Read the model definition and answer for the solid it produces. Units are mm, in the model's axes. A direction names the side the tool comes from. Coordinates: 2 decimals unless noted, no trailing zeros. Write each loop counter-clockwise with the first axis right and the second up, starting at its lowest first coordinate (ties: lowest second). Pieces come first, ordered by that corner, then holes. Notation, with made-up numbers: M -30.75,45 L 3.25,45 A18 cw 3.25,60 Z; hole C -26,20 d2. An arc over 180 degrees is marked long. Use a Markdown table: item, result. Add a question column.
Autodesk Inventor part; units mm, degrees
ref_plane "YZ Plane" through (0, 0, 0) normal (1, 0, 0) x (0, 1, 0)
ref_plane "XZ Plane" through (0, 0, 0) normal (0, 1, 0) x (-1, 0, 0)
ref_plane "XY Plane" through (0, 0, 0) normal (0, 0, 1) x (1, 0, 0)
sketch "Sketch1" plane through (0, 0, 0) normal (0, 1, 0) x (-1, 0, 0)
  line L0 (0, -3) -> (-0.5, -3)
  line L1 (-0.5, -3) -> (-0.5, -4.2634)
  line L2 (-0.5, -4.2634) -> (-0.5134, -4.2634)
  line L3 (-0.5134, -4.2634) -> (-4.9134, -3)
  line L4 (0, -3) -> (0, 0)
  line L5 (-4.9134, -3) -> (-4.9134, 0)
  line L6 (0, 0) -> (-4.9134, 0) construction
  line L7 (0, 3) -> (-0.5, 3)
  line L8 (-0.5, 3) -> (-0.5, 4.2634)
  line L9 (-0.5, 4.2634) -> (-0.5134, 4.2634)
  line L10 (-0.5134, 4.2634) -> (-4.9134, 3)
  line L11 (0, 3) -> (0, 0)
  line L12 (-4.9134, 3) -> (-4.9134, 0)
  dimension "d0" = 6
  dimension "d1" = 0.5
  dimension "d4" = 4.4
extrude "Extrusion1" add sketch "Sketch1" along normal blind 10
sketch "Sketch2" plane through (0, 0, -3) normal (-1, 0, 0) x (0, 0, 1)
  line L0 (3, 0) -> (3, 10) construction
  line L1 (0, 10) -> (6, 10)
  point P0 (3, 5)
hole "Hole2" at (0, 5, 0) direction (1, 0, 0) diameter 4.134 end through all
properties part number "m5_t_nut"
Item 1: Find section D-D on x = 1.85. Give the vertices of the cut face in (y, z), then the cut area to 3 significant figures.
Item 2: Each of these flat-tipped pins is pushed along its axis until it touches: pin 1 (0.6 mm diameter, centred on x = 0, y = 4.5, fed in from -Z); pin 2 (1.4 mm diameter, centred on y = 7, z = 4, fed in from -X); pin 3 (3.5 mm diameter, centred on y = 5, z = 0, fed in from +X). Where does it stop, or does it pass through?
Item 3: For faces 1 (the flat face through (0.5, 5, -4)), 2 (the flat face through (2.68, 4.93, 3.64)), 3 (the flat face through (0.5, 5, 4)), determine the directions among +Z, -Z, +X, -X, +Y, -Y from which every point of the face is accessible in a straight line to the end or side of a thin tool.
Item 4: Consider probe 1 along Y at (x, z) = (3.75, 0); probe 2 along Z at (x, y) = (0.4, 5.25); probe 3 along Z at (x, y) = (2.45, 5). Determine where each line is inside the solid, lowest interval first.
Item 5: Determine the mould class of faces 4 (the cylindrical face through (2.49, 2.95, -0.27)), 5 (the flat face through (0, 2.7, 0)), 6 (the flat face through (2, 0, 0)), 7 (the flat face through (2, 10, 0)) for opening direction Y: pulls with the +Y half, pulls with the -Y half, needs draft (parallel to the pull), parting line crosses it, or undercut.
Item 6: Find section B-B on z = 0. Give the vertices of the cut face in (x, y), then the cut area to 3 significant figures.
Geometry says:
| question | item | result |
|---|---|---|
| 1 | outline | M 0,-3.88 L 10,-3.88 L 10,3.88 L 0,3.88 Z; hole C 5,0 d4.13 |
| 1 | area | 64.2 mm2 |
| 2 | pin 1 | stops at z = -3 |
| 2 | pin 2 | stops at x = 0.5 |
| 2 | pin 3 | passes through |
| 3 | face 1 | -Z, -X, +Y, -Y |
| 3 | face 2 | +Z, +X, +Y, -Y |
| 3 | face 3 | +Z, -X, +Y, -Y |
| 4 | probe 1 | y = 0 to 2.93, 7.07 to 10 |
| 4 | probe 2 | z = -3 to -2.05, 2.05 to 3 |
| 4 | probe 3 | z = -3.71 to -2.07, 2.07 to 3.71 |
| 5 | face 4 | undercut |
| 5 | face 5 | needs draft |
| 5 | face 6 | pulls with the -Y half |
| 5 | face 7 | pulls with the +Y half |
| 6 | outline | M 0,0 L 4.91,0 L 4.91,2.93 L 0,2.93 Z; M 0,7.07 L 4.91,7.07 L 4.91,10 L 0,10 Z |
| 6 | area | 28.8 mm2 |
